Source: CAD feature listing. Evaluate the final solid. Frame: model axes, mm. A direction names the side the tool comes from. Give positions to 0.01 mm unless a question says otherwise; leave off trailing zeros. Order: outer loops, then holes, each group sorted by start corner. A loop starts at its lowest first (then second) coordinate and runs counter-clockwise, first axis right, second up. Notation, with made-up numbers: (13, 40.25) - (40, 40.25) arc R22 cw to (40, 70.25) - close; hole circle Ø4 at (38.5, 80.25). An arc over 180 degrees is marked (long way). Answer as CSV lines item,"result".
```python
from build123d import *

# Parameters (mm, degrees)
SKETCH4_W           = 64.77
SKETCH4_H           = 56.134
BOSS_EXTRUDE1_DEPTH = 19.05
CUT_EXTRUDE1_DEPTH  = 115.855093202
BOSS_EXTRUDE2_DEPTH = 19.05
SKETCH7_R           = 9.271
BOSS_EXTRUDE3_DEPTH = 25.4
FILLET1_R           = 6.35


with BuildPart() as part:
    # Sketch4 → Boss-Extrude1 (new body)
    with BuildSketch(Plane.XY):
        with Locations((-42.617275879, 56.806132071)):
            Rectangle(SKETCH4_W, SKETCH4_H)
    extrude(amount=BOSS_EXTRUDE1_DEPTH)

    # Sketch5 → Cut-Extrude1 (cut, through all)
    with BuildSketch(Plane.XY.offset(19.05)):
        Polygon((-74.321555879, 39.661132071), (-10.912995879, 39.661132071), (-10.912995879, 77.735732071), (-36.292675879, 77.735732071), (-36.292675879, 84.873132071), (-48.941875879, 84.873132071), (-48.941875879, 77.735732071), (-74.321555879, 77.735732071), align=None)
    extrude(amount=-CUT_EXTRUDE1_DEPTH, mode=Mode.SUBTRACT)

    # Sketch6 → Boss-Extrude2 (add)
    with BuildSketch(Plane.XZ.offset(-28.739132071)):
        Polygon((-42.617275879, 0), (-34.997275879, 0), (-34.997275879, 12.7), (-50.237275879, 12.7), (-50.237275879, 0), align=None)
    extrude(amount=BOSS_EXTRUDE2_DEPTH)

    # Sketch7 → Boss-Extrude3 (add)
    with BuildSketch(Plane(origin=(0, 0, 0), x_dir=(-1, 0, 0), z_dir=(0, 0, -1))):
        with Locations((42.617275879, 9.689132071)):
            Circle(SKETCH7_R)
    extrude(amount=-BOSS_EXTRUDE3_DEPTH)

    # Fillet1
    fillet1_edges = [part.edges().sort_by_distance(p)[0] for p in [
        (-50.237275879, 14.969950284, 6.35),
        (-42.617275879, 18.960132071, 12.7),
        (-34.997275879, 14.969950284, 6.35),
    ]]
    fillet(fillet1_edges, radius=FILLET1_R)


solid = part.part
```
(1) Access query for faces 1 (the cylindrical face through (-50.41, 15.2, 9.39)), 2 (the flat face through (-48.942, 81, 10)), 3 (the flat face through (-40, 38, 19.05)), 4 (the flat face through (-43, 39.661, 10)), 5 (the flat face through (-34.997, 23, 6)). Directions: +Z, -Z, +X, -X, +Y, -Y. A direction counts if a zero-diameter tool reaches every point of the face in a straight line with its end or side. Return the directions, or none.
Completed:
face 1,"+Z, -Z, -X"
face 2,"+Z, -Z, +Y"
face 3,"+Z, +X, -X, +Y"
face 4,"+Z, -Z"
face 5,"+Z, -Z, +X"
(2) Cut plane B-B (y = 50). Return loops of the section in (x, z).
Completed:
outline,"(-75, 0) - (-74.32, 0) - (-74.32, 19.05) - (-75, 19.05) - close; (-10.91, 0) - (-10.23, 0) - (-10.23, 19.05) - (-10.91, 19.05) - close"
(3) Cut plane D-D (z = 20). Return loops of the section in (x, y), then the cut area to 3 significant figures.
Completed:
outline,"circle Ø18.54 at (-42.62, 9.69)"
area,"270 mm²"
(4) Contact query for flat-ended pins moving along their axis: pin 1 (3.5 mm diameter, centred on y = 23, z = 4.5, fed in from +X); pin 2 (1.6 mm diameter, centred on x = -39.5, y = 25, fed in from +Z); pin 3 (8 mm diameter, centred on x = -24.5, z = 6, fed in from -Y). Output: stop coordinate, or through.
Completed:
pin 1,"x = -35"
pin 2,"z = 12.75"
pin 3,"y = 28.74"
(5) Mould query, pull axis Y, two halves, no side actions, for faces 6 (the flat face through (-23, 77.736, 10)), 7 (the flat face through (-75.002, 56, 9)), 8 (the flat face through (-62, 84.873, 9)). Classes: released by +Y, released by -Y, zero draft, split by the parting line, or undercut.
Completed:
face 6,"undercut"
face 7,"zero draft"
face 8,"released by +Y"
(6) Ray query, line 1 (X direction, y = 67, z = 10.5); line 2 (Y direction, x = -54.5, z = 8); line 3 (Y direction, x = -51, z = 8). Return the intervals inside material, ascending. Write a range as from..to.
Completed:
line 1,"-75..-74.32, -10.91..-10.23"
line 2,"28.74..39.66, 77.74..84.87"
line 3,"5.73..13.65, 28.74..39.66, 77.74..84.87"
(7) Cut plane C-C (z = 9.25). Return loops of the section in (x, y).
Completed:
outline,"(-75, 28.74) - (-50.24, 28.74) - (-50.24, 16.68) arc R6.35 cw to (-50.91, 13.84) arc R9.27 ccw (long way) to (-34.33, 13.84) arc R6.35 cw to (-35, 16.68) - (-35, 28.74) - (-10.23, 28.74) - (-10.23, 84.87) - (-36.29, 84.87) - (-36.29, 77.74) - (-10.91, 77.74) - (-10.91, 39.66) - (-74.32, 39.66) - (-74.32, 77.74) - (-48.94, 77.74) - (-48.94, 84.87) - (-75, 84.87) - close"
(8) Cut plane A-A (x = -18). Return loops of the section in (y, z), then the cut area to 3 significant figures.
Completed:
outline,"(28.74, 0) - (39.66, 0) - (39.66, 19.05) - (28.74, 19.05) - close; (77.74, 0) - (84.87, 0) - (84.87, 19.05) - (77.74, 19.05) - close"
area,"344 mm²"
